Design review of the part built by this model. Coordinates are the model's own, in mm. A direction names the side the tool comes from. Round coordinates to 2 decimals unless told otherwise and drop trailing zeros. Loops run counter-clockwise (first coordinate to the right, second up) from the corner with the lowest first, then second, coordinate; pieces in that order, holes last. Notation, with made-up numbers: (51.25, 5.25) - (101.25, 5.25) arc R8 cw to (101.25, 16.25) - close; hole circle Ø4 at (44.25, -30.75). An arc over 180 degrees is marked (long way). Answer as CSV lines item,"result". Start each with the question number.
(1) Consider section D-D (x = 11). Give the boundary of the cut face in (y, z), and give its area (3 significant figures).
(2) Consider section C-C (z = 15). Give the boundary of the cut face in (x, y), and give its area (3 significant figures).
(3) Consider section A-A (y = 0). Give the boundary of the cut face in (x, z).
(4) For P1, Ø1, axis at x = 6.5, z = 80.5, coming from the -Y side; P2, Ø10, axis at x = -3, y = -0.5, coming from the +Z side; P3, Ø3, axis at y = 9.5, z = 90, coming from the -X side; P4, Ø8, axis at x = -1.5, z = 40, coming from the -Y side, all flat-tipped, find the tip position at first contact; note any pin that passes through.
(5) Wall thickness on L1, parallel to Y at x = 0, z = 57; L2, parallel to Y at x = 0, z = 3.6; L3, parallel to Z at x = 11.75, y = 3: over which ranges is each line inside the solid? List them lowest first.
(6) Consider section B-B (x = 0). Give the boundary of the cut face in (y, z).
(7) For faces 1 (the flat face through (-12.2, 0.2, 5)), 2 (the flat face through (-5, 9, 115)), list the 3-axis set-ups (+Z, -Z, +X, -X, +Y, -Y) from which the entire face can be reached by the end or side of a thin tool; tool diameter is ignored.
from build123d import *

# Parameters (mm, degrees)
F0_W      = 27
F0_H      = 28
F1_DEPTH  = 5
F2_R      = 12
F2_R_2    = 10
F3_DEPTH  = 110
F3_FACE_R = 10
F4_DEPTH  = 5


with BuildPart() as f1:
    # F0 (on Top) → F1 (new body)
    with BuildSketch(Plane.XY):
        Rectangle(F0_W, F0_H)
    extrude(amount=F1_DEPTH)

    # F2 (on face) → F3 (join)
    with BuildSketch(Plane.XY.offset(5)):
        Circle(F2_R)
        Circle(F2_R_2, mode=Mode.SUBTRACT)
    extrude(amount=F3_DEPTH)

    # F3_face (on face) → F4 (cut, through all)
    with BuildSketch(Plane.XY.offset(5)):
        Circle(F3_FACE_R)
    extrude(amount=-F4_DEPTH, mode=Mode.SUBTRACT)


solid = f1.part
Determined:
1,outline,"(-14, 0) - (14, 0) - (14, 5) - (4.8, 5) - (4.8, 115) - (-4.8, 115) - (-4.8, 5) - (-14, 5) - close"
1,area,"1,200 mm^2"
2,outline,"circle Ø24 at (0, 0); hole circle Ø20 at (0, 0)"
2,area,"138 mm^2"
3,outline,"(-13.5, 0) - (-10, 0) - (-10, 115) - (-12, 115) - (-12, 5) - (-13.5, 5) - close; (10, 0) - (13.5, 0) - (13.5, 5) - (12, 5) - (12, 115) - (10, 115) - close"
4,P1,"stops at y = -10.39"
4,P2,"passes through"
4,P3,"stops at x = -8.94"
4,P4,"stops at y = -12"
5,L1,"y = -12 to -10, 10 to 12"
5,L2,"y = -14 to -10, 10 to 14"
5,L3,"z = 0 to 5"
6,outline,"(-14, 0) - (-10, 0) - (-10, 115) - (-12, 115) - (-12, 5) - (-14, 5) - close; (10, 0) - (14, 0) - (14, 5) - (12, 5) - (12, 115) - (10, 115) - close"
7,face 1,"+Z"
7,face 2,"+Z, +X, -X, +Y, -Y"
